Verification items for the finished model (mm, model axes). Face numbers are marked on the shaded views. A direction names the side the tool comes from. Give positions to 0.01 mm unless a question says otherwise; leave off trailing zeros. Order: outer loops, then holes, each group sorted by start corner. A loop starts at its lowest first (then second) coordinate and runs counter-clockwise, first axis right, second up. Notation, with made-up numbers: M -9.75,45.25 L 0.25,45.25 A27 ccw 0.25,73.25 Z; hole C -14.5,33.5 d4. An arc over 180 degrees is marked long. Answer as a JSON object with one key per item and string values.
```python
from build123d import *

# Parameters (mm, degrees)
BOSS_EXTRUDE1_DEPTH = 2.54
BOSS_EXTRUDE2_DEPTH = 2.54


with BuildPart() as part:
    # Sketch1 → Boss-Extrude1 (new body)
    with BuildSketch(Plane(origin=(0, 0, 0), x_dir=(1, 0, 0), z_dir=(0, 1, 0))):
        with BuildLine():
            Line((2.54, 0), (2.54, -22.098))
            ThreePointArc((2.54, -22.098), (0, -24.638), (-2.54, -22.098))
            Line((-2.54, -22.098), (-2.54, 0))
            ThreePointArc((-2.54, 0), (0, 2.54), (2.54, 0))
        make_face()
    extrude(amount=BOSS_EXTRUDE1_DEPTH)

    # Sketch2 → Boss-Extrude2 (add)
    with BuildSketch(Plane(origin=(0, 2.54, 0), x_dir=(1, 0, 0), z_dir=(0, 1, 0))):
        with BuildLine():
            ThreePointArc((-2.54, -22.098), (0, -24.638), (2.54, -22.098))
            ThreePointArc((2.54, -22.098), (0, -19.558), (-2.54, -22.098))
        make_face()
    extrude(amount=BOSS_EXTRUDE2_DEPTH)


solid = part.part
```
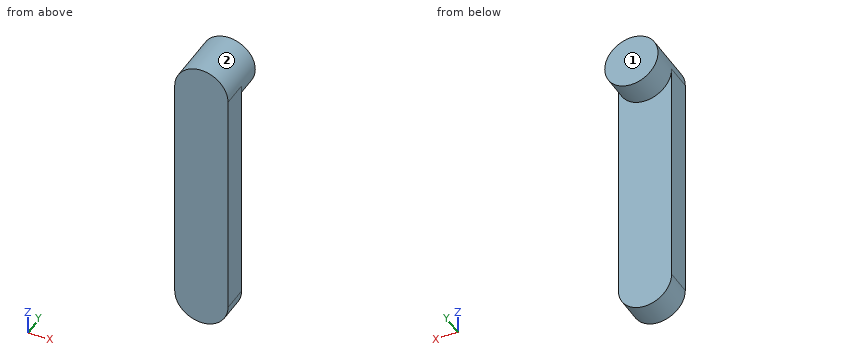
Q1. Gauge pin test, flat ends, axial feed: pin 1 Ø3 at (x, z) = (2, 2) entering from +Y; pin 2 Ø1.5 at (x, y) = (-1, 3) entering from -Z. Record the tip position at first contact, or that the pin passes through.
Resolved:
{"pin 1": "stops at y = 2.54", "pin 2": "stops at z = -2.51"}
Q2. Section check A-A on x = 0. Record the cut outline in (y, z).
Resolved:
{"outline": "M 0,-2.54 L 2.54,-2.54 L 2.54,19.56 L 5.08,19.56 L 5.08,24.64 L 0,24.64 Z"}
Q3. Section check B-B on y = 0.4. Record the cut outline in (x, z), then the cut area to 3 significant figures.
Resolved:
{"outline": "M -2.54,0 A2.54 ccw 2.54,0 L 2.54,22.1 A2.54 ccw -2.54,22.1 Z", "area": "133 mm²"}
Q4. Material ranges on L1, parallel to Y at x = -1.05, z = 5.5; L2, parallel to Z at x = -0.15, y = 2.2; L3, parallel to Z at x = 1.4, y = 1.15, recorded low to high.
Resolved:
{"L1": "y = 0 to 2.54", "L2": "z = -2.54 to 24.63", "L3": "z = -2.12 to 24.22"}
Q5. Tool access check on the marked faces 1 and 2. Record the directions out of +Z, -Z, +X, -X, +Y, -Y that give a thin tool (end or side, any length) a straight path to the whole face; none if there is none.
Resolved:
{"face 1": "+Z, -Z, +X, -X, +Y", "face 2": "+Y"}
Q6. Section check C-C on x = -2. Record the cut outline in (y, z), then the cut area to 3 significant figures.
Resolved:
{"outline": "M 0,-1.57 L 2.54,-1.57 L 2.54,20.53 L 5.08,20.53 L 5.08,23.66 L 0,23.66 Z", "area": "72.0 mm²"}
